Could you check a few things on this model? Use its own coordinates, in mm. Face numbers are marked on the shaded views. A direction names the side the tool comes from. Coordinates: 2 decimals unless noted, no trailing zeros. Loops run counter-clockwise (first coordinate to the right, second up) from the corner with the lowest first, then second, coordinate; pieces in that order, holes last. Notation, with made-up numbers: (53.5, 38.5) - (61.5, 38.5) arc R17 ccw to (61.5, 46.5) - close; hole circle Ø9 at (5, 55). An arc over 180 degrees is marked (long way). One line per item, written item: value. Start each with the question number.
(1) I'm going to push flat-ended pins straight in: P1, Ø10, axis at x = -203.5, z = 301, coming from the +Y side; P2, Ø10, axis at y = 110, z = 424.5, coming from the +X side; P3, Ø1, axis at x = -143, z = 193, coming from the +Y side. Where does each tip first touch, or does it pass through?
(2) If we section it at A-A on z = -836: Write out the boundary of the cut face in (x, y).
(3) If we section it at B-B on y = 295.5: Write out the boundary of the cut face in (x, z), then the cut area to 3 significant figures.
(4) If I drill on line 1 along Z through (x, y) = (185.5, 66.5); line 2 along X through (y, z) = (552, -724.5); line 3 along X through (y, z) = (270, -816.5), over which ranges is the centre line in solid material (lowest first)? Write a range as from..to.
(5) If we mould it in two halves opening along Z, with no side actions, what happens to the marked faces 1, 2, 3 and 4? For each: pulls with the +Z half, pulls with the -Z half, needs draft (parallel to the pull), parting line crosses it, or undercut.
(6) If we section it at C-C on x = -167.5: Write out the boundary of the cut face in (y, z).
(7) On a 3-axis mill with a long thin cutter (end or side, diameter ignored), from which of +Z, -Z, +X, -X, +Y, -Y can I reach the whole of each face in a straight line? I mean the marked faces 5 and 6. Say none if no direction works.
(8) If we section it at D-D on y = 427: Write out the boundary of the cut face in (x, z), then the cut area to 3 significant figures.
Autodesk Inventor part; units mm, degrees
ref_plane "YZ Plane" through (0, 0, 0) normal (1, 0, 0) x (0, 1, 0)
ref_plane "XZ Plane" through (0, 0, 0) normal (0, 1, 0) x (-1, 0, 0)
ref_plane "XY Plane" through (0, 0, 0) normal (0, 0, 1) x (1, 0, 0)
sketch "Sketch1" plane through (0, 0, 0) normal (0, 0, 1) x (1, 0, 0)
  line L0 (0, 0) -> (0, 800) construction
  line L1 (0, 800) -> (-75, 800)
  line L2 (-300, 0) -> (-300, 50)
  line L3 (-75, 800) -> (-118.3113, 400)
  line L4 (-118.3113, 400) -> (-300, 50)
  line L5 (0, 800) -> (75, 800)
  line L6 (300, 0) -> (300, 50)
  line L7 (75, 800) -> (118.3113, 400)
  line L8 (118.3113, 400) -> (300, 50)
  line L9 (300, 0) -> (-300, 0)
  dimension "d28" = 800
extrude "Extrusion1" add sketch "Sketch1" along normal mid plane 2000
sketch "Sketch5" plane through (-300, 0, 1000) normal (0, -1, 0) x (1, 0, 0)
  line L0 (0, -2000) -> (181.6887, -2000)
  line L1 (0, -2000) -> (0, 0)
  line L2 (100, -1900) -> (100, -100)
  line L3 (181.6887, -2000) -> (181.6887, 0)
  line L4 (100, -1900) -> (500, -1900)
  line L5 (600, -2000) -> (600, 0)
  line L6 (500, -1900) -> (500, -100)
  line L7 (500, -100) -> (100, -100)
  point P0 (300, -1000)
  dimension "d35" = 1800
extrude "Extrusion5" cut sketch "Sketch5" against normal blind 200
chamfer "Chamfer1" distance 130 angle 45 2 edges at (200, 200, 0) (-200, 200, 0)
sketch "Sketch6" plane through (-300, 200, 1000) normal (0, -1, 0) x (1, 0, 0)
  line L0 (370, -100) -> (370, -1900)
  line L1 (370, -100) -> (370, -1900)
  line L2 (230, -1900) -> (230, -100)
  line L3 (370, -1900) -> (230, -1900)
  line L4 (230, -1900) -> (230, -100)
  line L5 (230, -100) -> (370, -100)
  point P0 (300, -1000)
extrude "Extrusion6" cut sketch "Sketch6" against normal blind 400
sketch "Sketch7" plane through (200, 0, -900) normal (-1, 0, 0) x (0, 0, 1)
  line L0 (0, 0) -> (0, 70)
  line L1 (0, 0) -> (100, 0)
  line L2 (1800, 0) -> (0, 0)
  line L3 (100, 0) -> (100, 50)
  line L4 (100, 50) -> (200, 50)
  line L5 (200, 50) -> (200, 0)
  line L6 (200, 0) -> (100, 0)
  line L7 (1800, 0) -> (1700, 0)
  line L8 (1700, 0) -> (1700, 50)
  line L9 (1700, 50) -> (1600, 50)
  line L10 (1600, 50) -> (1600, 0)
  line L11 (1600, 0) -> (1700, 0)
  point P0 (900, 0)
  point P1 (200, 0)
  dimension "d43" = 100
  dimension "d44" = 50
  dimension "d45" = 100
  dimension "d46" = 50
  dimension "d47" = 100
  dimension "d48" = 50
  dimension "d49" = 100
  dimension "d50" = 50
sketch "Sketch8" plane through (-200, 0, 900) normal (1, 0, 0) x (0, 0, -1)
  line L0 (1800, 0) -> (0, 0)
  line L1 (1800, 0) -> (1700, 0)
  line L2 (1700, 0) -> (1700, 50)
  line L3 (1700, 50) -> (1600, 50)
  line L4 (1600, 50) -> (1600, 0)
  line L5 (0, 0) -> (100, 0)
  line L6 (100, 0) -> (100, 50)
  line L7 (100, 50) -> (200, 50)
  line L8 (200, 50) -> (200, 0)
  line L9 (200, 0) -> (100, 0)
  point P0 (900, 0)
  dimension "d55" = 100
  dimension "d56" = 50
  dimension "d57" = 100
  dimension "d58" = 50
  dimension "d59" = 100
  dimension "d60" = 50
  dimension "d61" = 100
  dimension "d62" = 50
extrude "Extrusion7" cut sketch "Sketch8" against normal blind 100
extrude "Extrusion8" cut sketch "Sketch7" against normal blind 100
properties part number "Jersey Curb" material "Concrete"
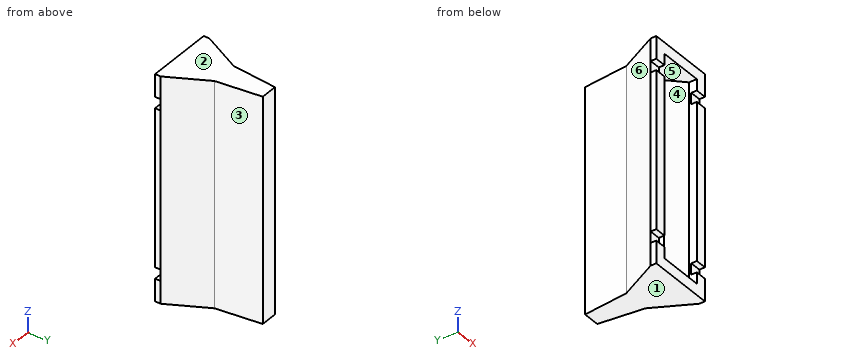
Values:
1. P1: stops at y = 245.53
1. P2: stops at x = 271.45
1. P3: stops at y = 353.4
2. outline: (-300, 0) - (-200, 0) - (-200, 70) - (-70, 200) - (-70, 600) - (70, 600) - (70, 200) - (200, 70) - (200, 0) - (300, 0) - (300, 50) - (118.31, 400) - (75, 800) - (-75, 800) - (-118.31, 400) - (-300, 50) - close
3. outline: (-172.56, -1000) - (172.56, -1000) - (172.56, 1000) - (-172.56, 1000) - close; hole (-70, -900) - (70, -900) - (70, 900) - (-70, 900) - close
3. area: 438,000 mm2
4. line 1: z = -1000..-900, 900..1000
4. line 2: x = -101.85..-70, 70..101.85
4. line 3: x = -185.8..-70, 70..185.8
5. face 1: pulls with the -Z half
5. face 2: pulls with the +Z half
5. face 3: needs draft
5. face 4: undercut
6. outline: (0, -1000) - (305.24, -1000) - (305.24, 1000) - (0, 1000) - (0, 900) - (102.5, 900) - (102.5, -900) - (0, -900) - close
7. face 5: -Y
7. face 6: +Z, -Z, -X, +Y
8. outline: (-115.39, -1000) - (115.39, -1000) - (115.39, 1000) - (-115.39, 1000) - close; hole (-70, -900) - (70, -900) - (70, 900) - (-70, 900) - close
8. area: 210,000 mm2
